from build123d import *

# Parameters (mm, degrees)
SKETCH_1_R      = 3.4
EXTRUDE_2_DEPTH = 7.6
SKETCH_2_W      = 6.529029983
SKETCH_2_H      = 6.008592339
EXTRUDE_5_DEPTH = 7.5
FILLET_1_R      = 0.8


with BuildPart() as part:
    # 草图1 → 凸台-拉伸2 (new body)
    with BuildSketch(Plane.XY):
        with BuildLine():
            Line((53.915690558, 12), (-21.801891992, 12))
            Line((-21.801891992, 12), (-21.801891992, 0))
            Line((-21.801891992, 0), (53.915690558, 0))
            ThreePointArc((53.915690558, 0), (55.600804493, 0.241494028), (57.150270111, 0.946536325))
            Line((57.150270111, 0.946536325), (57.150270111, 3.646811713))
            ThreePointArc((57.150270111, 3.646811713), (49.915690558, 6), (57.150270111, 8.353188287))
            Line((57.150270111, 8.353188287), (57.150270111, 11.053463675))
            ThreePointArc((57.150270111, 11.053463675), (55.600804493, 11.758505972), (53.915690558, 12))
        make_face()
        with Locations((-14.326955942, 6)):
            Circle(SKETCH_1_R, mode=Mode.SUBTRACT)
    extrude(amount=EXTRUDE_2_DEPTH)

    # 草图2 → 凸台-拉伸5 (add)
    with BuildSketch(Plane.XY.offset(7.6)):
        with Locations((-8.162440951, 7.229472235)):
            Rectangle(SKETCH_2_W, SKETCH_2_H)
    extrude(amount=-EXTRUDE_5_DEPTH)

    # 圆角1
    fillet_1_edges = [part.edges().sort_by_distance(p)[0] for p in [
        (57.150270111, 8.353188287, 3.8),
        (57.150270111, 3.646811713, 3.8),
    ]]
    fillet(fillet_1_edges, radius=FILLET_1_R)


solid = part.part
Could you check a few things on this model? Use its own coordinates, in mm. A direction names the side the tool comes from. Give positions to 0.01 mm unless a question says otherwise; leave off trailing zeros. Loops run counter-clockwise (first coordinate to the right, second up) from the corner with the lowest first, then second, coordinate; pieces in that order, holes last. Notation, with made-up numbers: M 42.25,-4.5 L 88.25,-4.5 A12 ccw 88.25,0.5 Z; hole C 12,-13.75 d7. An arc over 180 degrees is marked long. Answer as a JSON object with one key per item and string values.
Q1. For faces 1 (the flat face through (-11.427, 6, 4)), 2 (the flat face through (16, 0, 4)), which set-ups out of +Z, -Z, +X, -X, +Y, -Y let a thin tool reach every point of the face, with its end or its side?
Values found:
{"face 1": "+Z, -Z", "face 2": "+Z, -Z, +X, -X, -Y"}
Q2. Suppose I cut it at A-A, the plane y = 6. List the corners of the cut face in (x, z) for me, plus the area to 3 significant figures.
Values found:
{"outline": "M -21.8,0 L -17.73,0 L -17.73,7.6 L -21.8,7.6 Z; M -11.43,0.1 L -10.93,0.1 L -10.93,0 L 49.92,0 L 49.92,7.6 L -11.43,7.6 Z", "area": "497 mm²"}
Q3. Suppose I cut it at B-B, the plane x = 51. List the corners of the cut face in (y, z) for me, plus the area to 3 significant figures.
Values found:
{"outline": "M 0,0 L 3.26,0 L 3.26,7.6 L 0,7.6 Z; M 8.74,0 L 12,0 L 12,7.6 L 8.74,7.6 Z", "area": "49.6 mm²"}
Q4. If we mould it in two halves opening along Y, with no side actions, what happens to faces 3 (the cylindrical face through (55.624, 11.752, 3.747)), 4 (the cylindrical face through (-17.724, 6.149, 3.747)), 5 (the cylindrical face through (49.917, 5.882, 3.747)), 6 (the flat face through (17, 6, 7.6))? For each: pulls with the +Y half, pulls with the -Y half, needs draft (parallel to the pull), parting line crosses it, or undercut.
Values found:
{"face 3": "pulls with the +Y half", "face 4": "undercut", "face 5": "undercut", "face 6": "needs draft"}
Q5. If I drill on probe 1 along X at (y, z) = (6, 5.5); probe 2 along Y at (x, z) = (-13.5, 5.5); probe 3 along X at (y, z) = (8.5, 0.5), over which ranges is the centre line in solid material (lowest first)? Write a range as [from, to].
Values found:
{"probe 1": "x = [-21.8, -17.73], [-11.43, 49.92]", "probe 2": "y = [0, 2.7], [9.3, 12]", "probe 3": "x = [-21.8, -16.63], [-12.02, 50.79]"}
Q6. Suppose I cut it at C-C, the plane z = 2.5. List the corners of the cut face in (x, y) for me.
Values found:
{"outline": "M -21.8,0 L 53.92,0 A6 ccw 57.15,0.95 L 57.15,1.86 A0.8 ccw 55.94,2.55 A4 cw long 55.94,9.45 A0.8 ccw 57.15,10.14 L 57.15,11.05 A6 ccw 53.92,12 L -21.8,12 Z; hole M -11.43,4.23 L -11.43,7.77 A3.4 ccw long Z"}
